from build123d import *

# Parameters (mm, degrees)
F1_DEPTH = 6
F2_SIZE2 = 1.992278
F2_SIZE  = 2.55


with BuildPart() as f1:
    # F0 (on Top) → F1 (new body)
    with BuildSketch(Plane.XY):
        Polygon((3.464102, 2), (-3.464102, 2), (0, -4), align=None)
    extrude(amount=F1_DEPTH)

    # F2
    f2_edges = [f1.edges().sort_by_distance(p)[0] for p in [
        (1.732051, -1, 6),
        (-1.732051, -1, 6),
        (0, 2, 6),
    ]]
    chamfer(f2_edges, length=F2_SIZE, length2=F2_SIZE2)


solid = f1.part
For this review, take the finished solid that the model builds, in its own axes (mm). Round coordinates to 2 decimals unless told otherwise and drop trailing zeros. Loops run counter-clockwise (first coordinate to the right, second up) from the corner with the lowest first, then second, coordinate; pieces in that order, holes last. Notation, with made-up numbers: (0.5, -27.5) - (10.5, -27.5) arc R22 cw to (10.5, 0.5) - close; hole circle Ø5 at (24.25, -38.5). An arc over 180 degrees is marked (long way). Put each result on its own line as item: value. Start each with the question number.
1. Consider section C-C on y = -2.75. State the section outline as (x, z) points, plus the area to 3 significant figures.
2. Consider section B-B on x = -2.25. State the section outline as (y, z) points, plus the area to 3 significant figures.
3. For probe 1 along Z at (x, y) = (-3, 1.25); probe 2 along Y at (x, z) = (-1, 5); probe 3 along Y at (x, z) = (2.75, 2.5), list the stretches that pass through material, from the lowest coordinate up. Write a range as [from, to].
4. Consider section D-D on y = 0.5. State the section outline as (x, z) points, plus the area to 3 significant figures.
5. Consider section A-A on z = 1. State the section outline as (x, y) points, plus the area to 3 significant figures.
6. Insertion check: P1, Ø1, axis at x = 2, z = 4, coming from the +Y side; P2, Ø1, axis at y = -0.5, z = 5, coming from the -X side; P3, Ø1.5, axis at y = -2.5, z = 4.5, coming from the -X side. Each pin has a flat end and moves straight along its axis. Give the tip position at first contact, or say it passes through.
Result sheet:
1. outline: (-0.72, 0) - (0.72, 0) - (0.72, 3.45) - (0, 4.25) - (-0.72, 3.45) - close
1. area: 5.56 mm^2
2. outline: (-0.1, 0) - (2, 0) - (2, 3.45) - (1.3, 4.35) - (-0.1, 3.45) - close
2. area: 8.20 mm^2
3. probe 1: [0, 3.48]
3. probe 2: [0.15, 0.79]
3. probe 3: [0.76, 2]
4. outline: (-2.6, 0) - (2.6, 0) - (2.6, 3.45) - (0.87, 5.37) - (-0.87, 5.37) - (-2.6, 3.45) - close
4. area: 24.6 mm^2
5. outline: (-3.46, 2) - (0, -4) - (3.46, 2) - close
5. area: 20.8 mm^2
6. P1: y = 1.96
6. P2: x = -1.16
6. P3: x = -0.72
